```python
from build123d import *

# Parameters (mm, degrees)
F1_DEPTH = 2.5
F2_R     = 2.49999


# Not quite as in the source:
# - a fillet or chamfer is up to 0.001 mm smaller than in the source, because OpenCascade refuses the exact size


with BuildPart() as f1:
    # F0 (on Front) → F1 (new body, symmetric)
    with BuildSketch(Plane.XZ):
        with BuildLine():
            ThreePointArc((23.5, -4.8265362185), (16.6678157232, 11.6678157232), (0.1734637815, 18.5))
            Line((0.1734637815, 18.5), (-0.1734637815, 18.5))
            ThreePointArc((-0.1734637815, 18.5), (-16.6678157232, 11.6678157232), (-23.5, -4.8265362185))
            Line((-23.5, -4.8265362185), (-23.5, -11.6431219986))
            ThreePointArc((-23.5, -11.6431219986), (-21.4916669312, -16.4916669312), (-16.6431219986, -18.5))
            Line((-16.6431219986, -18.5), (16.6431219986, -18.5))
            ThreePointArc((16.6431219986, -18.5), (21.4916669312, -16.4916669312), (23.5, -11.6431219986))
            Line((23.5, -11.6431219986), (23.5, -4.8265362185))
        make_face()
        with BuildLine():
            Line((-0.1734637815, 13.4999999712), (0.1734637815, 13.4999999712))
            ThreePointArc((0.1734637815, 13.4999999712), (13.1322817969, 8.1322817969), (18.4999999712, -4.8265362185))
            Line((18.4999999712, -4.8265362185), (18.4999999712, -11.6431219986))
            ThreePointArc((18.4999999712, -11.6431219986), (17.9561330049, -12.9561330049), (16.6431219986, -13.4999999712))
            Line((16.6431219986, -13.4999999712), (-16.6431219986, -13.4999999712))
            ThreePointArc((-16.6431219986, -13.4999999712), (-17.9561330049, -12.9561330049), (-18.4999999712, -11.6431219986))
            Line((-18.4999999712, -11.6431219986), (-18.4999999712, -4.8265362185))
            ThreePointArc((-18.4999999712, -4.8265362185), (-13.1322817969, 8.1322817969), (-0.1734637815, 13.4999999712))
        make_face(mode=Mode.SUBTRACT)
    extrude(amount=F1_DEPTH, both=True)

    # F2 (radius 2.5 in the source; OpenCascade refuses exactly that, so slightly less here)
    f2_edges = [f1.edges().sort_by_distance(p)[0] for p in [
        (21.491667, 2.5, -16.491667),
        (23.5, 2.5, -8.234829),
        (16.667816, 2.5, 11.667816),
        (0, 2.5, 18.5),
        (-16.667816, 2.5, 11.667816),
        (-23.5, 2.5, -8.234829),
        (-21.491667, 2.5, -16.491667),
        (0, 2.5, -18.5),
        (0, 2.5, 13.5),
        (13.132282, 2.5, 8.132282),
        (18.5, 2.5, -8.234829),
        (17.956133, 2.5, -12.956133),
        (0, 2.5, -13.5),
        (-17.956133, 2.5, -12.956133),
        (-18.5, 2.5, -8.234829),
        (-13.132282, 2.5, 8.132282),
        (21.491667, -2.5, -16.491667),
        (23.5, -2.5, -8.234829),
        (16.667816, -2.5, 11.667816),
        (0, -2.5, 18.5),
        (-16.667816, -2.5, 11.667816),
        (-23.5, -2.5, -8.234829),
        (-21.491667, -2.5, -16.491667),
        (0, -2.5, -18.5),
        (0, -2.5, 13.5),
        (13.132282, -2.5, 8.132282),
        (18.5, -2.5, -8.234829),
        (17.956133, -2.5, -12.956133),
        (0, -2.5, -13.5),
        (-17.956133, -2.5, -12.956133),
        (-18.5, -2.5, -8.234829),
        (-13.132282, -2.5, 8.132282),
    ]]
    fillet(f2_edges, radius=F2_R)


solid = f1.part
```
Part model, mm, in its own coordinate system. A direction names the side the tool comes from. Coordinates: 2 decimals unless noted, no trailing zeros. Order: outer loops, then holes, each group sorted by start corner. A loop starts at its lowest first (then second) coordinate and runs counter-clockwise, first axis right, second up. Notation, with made-up numbers: (18, 16) -> (57, 16) arc R21 ccw to (57, 46) -> close; hole circle Ø10 at (28, -6.5). An arc over 180 degrees is marked (long way). Put each result on its own line as item: value. Start each with the question number.
(1) Probe line 1 along X through (y, z) = (-1, 11); line 2 along X through (y, z) = (-0.1, 12); line 3 along Z through (x, y) = (-13.5, -0.5). List the from-to ranges inside material, lowest first. Write a range as [from, to].
(2) Mould opens along Z. For faces 4 (the face through (0.233, -1.748, -17.787)), 5 (the face through (-0.233, 1.748, -14.213)), 6 (the face through (22.787, 1.748, -8.187)) say: pulls with the +Z half, pulls with the -Z half, needs draft (parallel to the pull), parting line crosses it, or undercut.
(3) Band-saw the part on C-C (y = 0.7). Give the cut face in (x, z).
(4) Band-saw the part on A-A (y = -1.5). Give the cut face in (x, z), then the cut area to 3 significant figures.
(5) Which spindle directions (+Z, -Z, +X, -X, +Y, -Y) get a long thin tool onto all of the face, cutting with end or side? Do faces 1 (the face through (22.787, -1.748, -8.187)), 2 (the face through (-19.252, -1.787, -8.187)), 3 (the face through (-19.213, 1.748, -8.187)). Say none if no direction does.
Determined:
1. line 1: x = [-17.02, -9.82], [9.82, 17.02]
1. line 2: x = [-16.33, -7.44], [7.44, 16.33]
1. line 3: z = [-18.45, -13.55], [7.83, 14.26]
2. face 4: pulls with the -Z half
2. face 5: undercut
2. face 6: needs draft
3. outline: (-23.4, -11.64) arc R6.76 ccw to (-16.64, -18.4) -> (16.64, -18.4) arc R6.76 ccw to (23.4, -11.64) -> (23.4, -4.83) arc R23.23 ccw to (0.17, 18.4) -> (-0.17, 18.4) arc R23.23 ccw to (-23.4, -4.83) -> close; hole (-18.6, -11.64) arc R1.96 ccw to (-16.64, -13.6) -> (16.64, -13.6) arc R1.96 ccw to (18.6, -11.64) -> (18.6, -4.83) arc R18.43 ccw to (0.17, 13.6) -> (-0.17, 13.6) arc R18.43 ccw to (-18.6, -4.83) -> close
4. outline: (-23, -11.64) arc R6.36 ccw to (-16.64, -18) -> (16.64, -18) arc R6.36 ccw to (23, -11.64) -> (23, -4.83) arc R22.83 ccw to (0.17, 18) -> (-0.17, 18) arc R22.83 ccw to (-23, -4.83) -> close; hole (-19, -11.64) arc R2.36 ccw to (-16.64, -14) -> (16.64, -14) arc R2.36 ccw to (19, -11.64) -> (19, -4.83) arc R18.83 ccw to (0.17, 14) -> (-0.17, 14) arc R18.83 ccw to (-19, -4.83) -> close
4. area: 506 mm²
5. face 1: +Z, -Z, +X, -Y
5. face 2: -Y
5. face 3: +Y
